from build123d import *

# Parameters (mm, degrees)
SKETCH1_W           = 139.7
SKETCH1_H           = 50.8
BOSS_EXTRUDE1_DEPTH = 6.35
SKETCH2_W           = 12.7
SKETCH2_H           = 6.35
BOSS_EXTRUDE2_DEPTH = 6.35
CUT_EXTRUDE1_DEPTH  = 6.35
CUT_EXTRUDE8_DEPTH  = 6.35
CUT_EXTRUDE2_DEPTH  = 6.35
SKETCH5_R           = 1.504
CUT_EXTRUDE6_DEPTH  = 6.35
SKETCH6_R           = 6
CUT_EXTRUDE7_DEPTH  = 6.35


with BuildPart() as part:
    # Sketch1 → Boss-Extrude1 (new body)
    with BuildSketch(Plane.XY):
        Rectangle(SKETCH1_W, SKETCH1_H)
    extrude(amount=BOSS_EXTRUDE1_DEPTH)

    # Sketch2 → Boss-Extrude2 (add)
    with BuildSketch(Plane(origin=(0, 0, 0), x_dir=(-1, 0, 0), z_dir=(0, 0, -1))):
        with Locations((-57.15, -28.575)):
            Rectangle(SKETCH2_W, SKETCH2_H)
        with Locations((-25.4, 28.575)):
            Rectangle(SKETCH2_W, SKETCH2_H)
    boss_extrude2 = extrude(amount=-BOSS_EXTRUDE2_DEPTH)

    # Sketch3 → Cut-Extrude1 (cut)
    with BuildSketch(Plane(origin=(0, 0, 0), x_dir=(-1, 0, 0), z_dir=(0, 0, -1))):
        Polygon((-46.5455, -25.4), (-46.5455, -15.875), (-49.53, -15.875), (-49.53, -12.7), (-46.5455, -12.7), (-46.5455, -11.1125), (-42.3545, -11.1125), (-42.3545, -12.7), (-39.37, -12.7), (-39.37, -15.875), (-42.3545, -15.875), (-42.3545, -25.4), align=None)
    cut_extrude1 = extrude(amount=-CUT_EXTRUDE1_DEPTH, mode=Mode.SUBTRACT)

    # Sketch7 → Cut-Extrude8 (cut)
    with BuildSketch(Plane(origin=(0, 0, 0), x_dir=(-1, 0, 0), z_dir=(0, 0, -1))):
        Polygon((-38.1, 25.4), (-69.85, -19.05), (-69.85, 25.4), align=None)
    cut_extrude8 = extrude(amount=-CUT_EXTRUDE8_DEPTH, mode=Mode.SUBTRACT)

    # Mirror2: Boss-Extrude2, Cut-Extrude8 across plane
    add(boss_extrude2.mirror(Plane(origin=(0, 0, 0), x_dir=(0, 0, 1), z_dir=(1, 0, 0))))
    add(cut_extrude8.mirror(Plane(origin=(0, 0, 0), x_dir=(0, 0, 1), z_dir=(1, 0, 0))), mode=Mode.SUBTRACT)

    # Mirror4: Cut-Extrude1 across plane
    add(cut_extrude1.mirror(Plane(origin=(0, 0, 0), x_dir=(0, 0, 1), z_dir=(1, 0, 0))), mode=Mode.SUBTRACT)

    # Sketch4 → Cut-Extrude2 (cut)
    with BuildSketch(Plane(origin=(0, 0, 0), x_dir=(-1, 0, 0), z_dir=(0, 0, -1))):
        Polygon((2.0955, 25.4), (-2.0955, 25.4), (-2.0955, 15.875), (-5.08, 15.875), (-5.08, 12.7), (-2.0955, 12.7), (-2.0955, 11.1125), (2.0955, 11.1125), (2.0955, 12.7), (5.08, 12.7), (5.08, 15.875), (2.0955, 15.875), align=None)
    extrude(amount=-CUT_EXTRUDE2_DEPTH, mode=Mode.SUBTRACT)

    # Sketch5 → Cut-Extrude6 (cut)
    with BuildSketch(Plane(origin=(0, 0, 0), x_dir=(-1, 0, 0), z_dir=(0, 0, -1))):
        with Locations((-7.75, 6.423393759)):
            Circle(SKETCH5_R)
        with Locations((-15.5, -7)):
            Circle(SKETCH5_R)
        with Locations((-7.75, -20.423393759)):
            Circle(SKETCH5_R)
        with Locations((7.75, -20.423393759)):
            Circle(SKETCH5_R)
        with Locations((15.5, -7)):
            Circle(SKETCH5_R)
        with Locations((7.75, 6.423393759)):
            Circle(SKETCH5_R)
    extrude(amount=-CUT_EXTRUDE6_DEPTH, mode=Mode.SUBTRACT)

    # Sketch6 → Cut-Extrude7 (cut)
    with BuildSketch(Plane(origin=(0, 0, 0), x_dir=(-1, 0, 0), z_dir=(0, 0, -1))):
        with Locations((0, -14)):
            Circle(SKETCH6_R)
    extrude(amount=-CUT_EXTRUDE7_DEPTH, mode=Mode.SUBTRACT)


solid = part.part
The listing builds one solid part. Answer for the finished solid, in the listing's coordinates (mm). A direction names the side the tool comes from. Coordinates: 2 decimals unless noted, no trailing zeros. Loops run counter-clockwise (first coordinate to the right, second up) from the corner with the lowest first, then second, coordinate; pieces in that order, holes last. Notation, with made-up numbers: (-17, 61) -> (3, 61) arc R34 cw to (3, 99) -> close; hole circle Ø5 at (-16.5, 86). An arc over 180 degrees is marked (long way). Write item = value, one per line. Start each with the question number.
1) A cutting plane is placed at A-A (x = -15.5). Give the vertices of the cut face in (y, z), then the cut area to 3 significant figures.
2) The mould has two halves that part along X. Classify faces 6 (the face through (-49.53, -14, 3)), 7 (the face through (53.75, 3.49, 3.13)), 8 (the face through (67, -25.4, 3)): released by +X, released by -X, zero draft, split by the parting line, or undercut.
3) Straight lines are drawn through the part: line 1 (Y direction, x = -7.75, z = 2.75); line 2 (Y direction, x = -15.5, z = 3); line 3 (X direction, y = 28.5, z = 4). For each, find the intervals that lie inside material, in ascending order. Write a range as from..to.
4) A cutting plane is placed at D-D (z = 1.5). Count the separate pieces of the cut face and the enclosed holes in it, then the cut area to 3 significant figures.
5) Given pin 1 Ø2 at (x, z) = (0.5, 2.5) entering from +Y; pin 2 Ø0.9 at (x, z) = (41.5, 3.5) entering from -Y; pin 3 Ø1 at (y, z) = (14.5, 3) entering from +X, each flat-ended and moving along its own axis, determine where each tip first touches the part or whether it passes through.
6) A cutting plane is placed at C-C (x = 44). Give the vertices of the cut face in (y, z), then the cut area to 3 significant figures.
7) A cutting plane is placed at B-B (y = 24). Give the vertices of the cut face in (x, z), then the cut area to 3 significant figures.
8) A tool of negligible diameter and unlimited length cuts with its end or side. For faces 1 (the face through (-44, -11.112, 3)), 2 (the face through (-11, 25.4, 3)), 3 (the face through (35, 25.4, 3)), 4 (the face through (-5.08, 14, 3)), 5 (the face through (69.85, -22, 3)), from which of +Z, -Z, +X, -X, +Y, -Y can it reach the whole face along a straight path? Write none if from no direction.
Responses:
q1.outline = (-25.4, 0) -> (-8.5, 0) -> (-8.5, 6.35) -> (-25.4, 6.35) -> close; (-5.5, 0) -> (25.4, 0) -> (25.4, 6.35) -> (-5.5, 6.35) -> close
q1.area = 303 mm²
q2.face_6 = undercut
q2.face_7 = released by +X
q2.face_8 = zero draft
q3.line_1 = -25.4..-21.93, -18.92..4.92, 7.93..25.4
q3.line_2 = -25.4..-8.5, -5.5..25.4
q3.line_3 = -31.75..-19.05, 19.05..31.75
q4.separate_pieces = 1
q4.enclosed_holes = 7
q4.area = 5,620 mm²
q5.pin_1 = 11.11
q5.pin_2 = -25.4
q5.pin_3 = 46.24
q6.outline = (-11.11, 0) -> (17.14, 0) -> (17.14, 6.35) -> (-11.11, 6.35) -> close
q6.area = 179 mm²
q7.outline = (-39.1, 0) -> (-2.1, 0) -> (-2.1, 6.35) -> (-39.1, 6.35) -> close; (2.1, 0) -> (39.1, 0) -> (39.1, 6.35) -> (2.1, 6.35) -> close
q7.area = 470 mm²
q8.face_1 = +Z, -Z, -Y
q8.face_2 = +Z, -Z, +Y
q8.face_3 = +Z, -Z, +X, +Y
q8.face_4 = +Z, -Z
q8.face_5 = +Z, -Z, +X, +Y, -Y
